from build123d import *

# Parameters (mm, degrees)
BOSS_EXTRUDE1_DEPTH = 30
SKETCH3_R           = 1.5
CUT_EXTRUDE1_DEPTH  = 7.5
SKETCH6_W           = 27
SKETCH6_H           = 13.5
CUT_EXTRUDE2_DEPTH  = 6


with BuildPart() as part:
    # Sketch1 → Boss-Extrude1 (new body)
    with BuildSketch(Plane.XY):
        Polygon((0, 0), (21.940611049, 0), (0, 20.459950802), align=None)
    extrude(amount=-BOSS_EXTRUDE1_DEPTH)

    # Sketch3 → Cut-Extrude1 (cut)
    with BuildSketch(Plane.XZ):
        with Locations((11.940611049, -15)):
            Circle(SKETCH3_R)
    extrude(amount=-CUT_EXTRUDE1_DEPTH, mode=Mode.SUBTRACT)

    # Sketch6 → Cut-Extrude2 (cut)
    with BuildSketch(Plane.ZY):
        with Locations((-15, 6.75)):
            Rectangle(SKETCH6_W, SKETCH6_H)
    extrude(amount=-CUT_EXTRUDE2_DEPTH, mode=Mode.SUBTRACT)


solid = part.part
Here's how the part is built. I have some questions about the finished solid (model axes, mm). A direction names the side the tool comes from. Round coordinates to 2 decimals unless told otherwise and drop trailing zeros. Order: outer loops, then holes, each group sorted by start corner. A loop starts at its lowest first (then second) coordinate and runs counter-clockwise, first axis right, second up. Notation, with made-up numbers: M 52,-26.5 L 93,-26.5 A31 ccw 93,1.5 Z; hole C 82.25,25.5 d9. An arc over 180 degrees is marked long. Return JSON: item names as keys, results as strings. Group by question number.
1. If we mould it in two halves opening along Z, with no side actions, what happens to faces 1 (the face through (16, 0, -15)), 2 (the face through (6, 6, 0)), 3 (the face through (3, 7, -28.5))? For each: pulls with the +Z half, pulls with the -Z half, needs draft (parallel to the pull), parting line crosses it, or undercut.
2. On a 3-axis mill with a long thin cutter (end or side, diameter ignored), from which of +Z, -Z, +X, -X, +Y, -Y can I reach the whole of each face in a straight line? I mean faces 4 (the face through (10.442, 3.698, -14.934)), 5 (the face through (6, 6, -30)), 6 (the face through (3, 7, -1.5)). Say none if no direction works.
3. I'm going to push flat-ended pins straight in: pin 1 Ø3 at (x, z) = (2, -10) entering from -Y; pin 2 Ø1 at (x, z) = (10.5, -11.5) entering from +Y; pin 3 Ø6 at (x, z) = (11, -21) entering from +Y. Where does each tip first touch, or does it pass through?
4. If we section it at C-C on y = 6.5: List the corners of the cut face in (x, z) for me.
5. If we section it at D-D on y = 9.75: List the corners of the cut face in (x, z) for me.
6. Please list where these lines run through material, in increasing order: probe 1 along Z at (x, y) = (2, 10.5); probe 2 along Y at (x, z) = (9, -5); probe 3 along Y at (x, z) = (1, -4.5).
7. If we section it at A-A on z = -15: List the corners of the cut face in (x, y) for me, then the cut area to 3 significant figures.
8. If we section it at B-B on x = 11.25: List the corners of the cut face in (y, z) for me.
Reply:
{
 "1": {"face 1": "needs draft", "face 2": "pulls with the +Z half", "face 3": "undercut"},
 "2": {"face 4": "-Y", "face 5": "-Z, +X, -X, +Y, -Y", "face 6": "-X, -Y"},
 "3": {"pin 1": "y = 13.5", "pin 2": "y = 11.13", "pin 3": "y = 13"},
 "4": {"outline": "M 0,-30 L 14.97,-30 L 14.97,0 L 0,0 L 0,-1.5 L 6,-1.5 L 6,-28.5 L 0,-28.5 Z; hole C 11.94,-15 d3"},
 "5": {"outline": "M 0,-30 L 11.49,-30 L 11.49,0 L 0,0 L 0,-1.5 L 6,-1.5 L 6,-28.5 L 0,-28.5 Z"},
 "6": {"probe 1": "-30 to -28.5, -1.5 to 0", "probe 2": "0 to 12.07", "probe 3": "13.5 to 19.53"},
 "7": {"outline": "M 0,13.5 L 6,13.5 L 6,0 L 10.44,0 L 10.44,7.5 L 13.44,7.5 L 13.44,0 L 21.94,0 L 0,20.46 Z", "area": "121 mm^2"},
 "8": {"outline": "M 0,-30 L 9.97,-30 L 9.97,0 L 0,0 L 0,-13.67 L 7.5,-13.67 L 7.5,-16.33 L 0,-16.33 Z"}
}
